Here's how the part is built. I have some questions about the finished solid (model axes, mm). Give positions to 0.01 mm unless a question says otherwise; leave off trailing zeros. Order: outer loops, then holes, each group sorted by start corner. A loop starts at its lowest first (then second) coordinate and runs counter-clockwise, first axis right, second up. Notation, with made-up numbers: (42.25, 65.25) - (59.25, 65.25) arc R10 cw to (59.25, 74.25) - close; hole circle Ø7 at (70.5, 20.25). An arc over 180 degrees is marked (long way). One line per question, with ' | ' between items.
from build123d import *

# Parameters (mm, degrees)
SKETCH2_W               = 163.1
SKETCH2_H               = 171.98
SKETCH2_R               = 2.5527
SKETCH2_R_2             = 1.5875
BOSS_EXTRUDE2_DEPTH     = 1.5875
FILLET1_R               = 1
CUT_EXTRUDE1_DEPTH      = 238.715061694
CUT_EXTRUDE1_DEPTH_BACK = 238.715061694
SKETCH3_R               = 1.725


with BuildPart() as part:
    # Sketch2 → Boss-Extrude2 (new body)
    with BuildSketch(Plane.XY):
        with Locations((82.55, -85.99)):
            Rectangle(SKETCH2_W, SKETCH2_H)
        with Locations((82.55, -85)):
            Circle(SKETCH2_R, mode=Mode.SUBTRACT)
        with Locations((82.55, -169.48)):
            Circle(SKETCH2_R_2, mode=Mode.SUBTRACT)
        with Locations((4.7625, -169.48)):
            Circle(SKETCH2_R_2, mode=Mode.SUBTRACT)
        with Locations((31.75, -169.48)):
            Circle(SKETCH2_R_2, mode=Mode.SUBTRACT)
        with Locations((57.15, -169.48)):
            Circle(SKETCH2_R_2, mode=Mode.SUBTRACT)
        with Locations((6.35, -94.25)):
            Circle(SKETCH2_R_2, mode=Mode.SUBTRACT)
        with Locations((6.35, -68.85)):
            Circle(SKETCH2_R_2, mode=Mode.SUBTRACT)
        with Locations((6.35, -43.45)):
            Circle(SKETCH2_R_2, mode=Mode.SUBTRACT)
        with Locations((6.35, -18.05)):
            Circle(SKETCH2_R_2, mode=Mode.SUBTRACT)
        with Locations((19.05, -3.175)):
            Circle(SKETCH2_R_2, mode=Mode.SUBTRACT)
        with Locations((44.45, -3.175)):
            Circle(SKETCH2_R_2, mode=Mode.SUBTRACT)
        with Locations((69.85, -3.175)):
            Circle(SKETCH2_R_2, mode=Mode.SUBTRACT)
        with Locations((158.75, -43.45)):
            Circle(SKETCH2_R_2, mode=Mode.SUBTRACT)
        with Locations((158.75, -18.05)):
            Circle(SKETCH2_R_2, mode=Mode.SUBTRACT)
        with Locations((146.05, -3.175)):
            Circle(SKETCH2_R_2, mode=Mode.SUBTRACT)
        with Locations((107.95, -169.48)):
            Circle(SKETCH2_R_2, mode=Mode.SUBTRACT)
        with Locations((133.35, -169.48)):
            Circle(SKETCH2_R_2, mode=Mode.SUBTRACT)
        with Locations((160.3375, -169.48)):
            Circle(SKETCH2_R_2, mode=Mode.SUBTRACT)
        with Locations((158.75, -94.25)):
            Circle(SKETCH2_R_2, mode=Mode.SUBTRACT)
        with Locations((158.75, -68.85)):
            Circle(SKETCH2_R_2, mode=Mode.SUBTRACT)
        with Locations((95.25, -3.175)):
            Circle(SKETCH2_R_2, mode=Mode.SUBTRACT)
        with Locations((120.65, -3.175)):
            Circle(SKETCH2_R_2, mode=Mode.SUBTRACT)
    extrude(amount=BOSS_EXTRUDE2_DEPTH)

    # Fillet1
    fillet1_edges = [part.edges().sort_by_distance(p)[0] for p in [
        (1, -171.98, 0.79375),
        (1, 0, 0.79375),
        (164.1, 0, 0.79375),
        (164.1, -171.98, 0.79375),
    ]]
    fillet(fillet1_edges, radius=FILLET1_R)

    # Sketch3 → Cut-Extrude1 (cut, two sides: drawn at the far end of the back side and taken through both)
    with BuildSketch(Plane.XY.offset(1.5875).offset(-CUT_EXTRUDE1_DEPTH_BACK)):
        with Locations((42.55, -108.63038)):
            Circle(SKETCH3_R)
        with Locations((82.55, -108.63038)):
            Circle(SKETCH3_R)
        with Locations((122.55, -108.63038)):
            Circle(SKETCH3_R)
        with Locations((42.55, -118.63038)):
            Circle(SKETCH3_R)
        with Locations((82.55, -118.63038)):
            Circle(SKETCH3_R)
        with Locations((122.55, -118.63038)):
            Circle(SKETCH3_R)
    extrude(amount=CUT_EXTRUDE1_DEPTH + CUT_EXTRUDE1_DEPTH_BACK, mode=Mode.SUBTRACT)


solid = part.part
1) Please list where these lines run through material, in increasing order: L1, parallel to X at y = -68.85, z = 0.5; L2, parallel to Y at x = 95.25, z = 0.65; L3, parallel to X at y = -86, z = 1.3.
Model answer:
L1: x = 1 to 4.76, 7.94 to 157.16, 160.34 to 164.1 | L2: y = -171.98 to -4.76, -1.59 to 0 | L3: x = 1 to 80.2, 84.9 to 164.1
2) Thinking about a two-plate mould opening in X: for faces 1 (the face through (100, -85, 1.588)), 2 (the face through (83.728, -87.265, 0.783)), which applies, +X half, -X half, draft (parallel to the pull), parting line (faces both ways), or undercut?
Model answer:
face 1: draft | face 2: undercut
3) I want a section at A-A (y = -85). List the corners of the cut face in (x, z) for me, plus the area to 3 significant figures.
Model answer:
outline: (1, 0) - (80, 0) - (80, 1.59) - (1, 1.59) - close; (85.1, 0) - (164.1, 0) - (164.1, 1.59) - (85.1, 1.59) - close | area: 251 mm2
